```python
from build123d import *

# Parameters (mm, degrees)
F3_D = 15


with BuildPart() as f1:
    # F0 (on Right) → F1 (revolve)
    with BuildSketch(Plane.YZ):
        Polygon((-31.213203, 0), (0, 0), (0, 30), (-5, 30), (-15.606602, 19.393398), (-26.213203, 30), (-31.213203, 30), align=None)
    revolve(axis=Axis((0, -15.606602, 0), (0, 1, 0)))

    # F3 (through all)
    with Locations(Plane(origin=(0, 0, 0), x_dir=(1, 0, 0), z_dir=(0, 1, 0))):
        with Locations((0, 0)):
            Hole(F3_D / 2)


solid = f1.part
```
Work out the finished part from the listing and answer in its coordinate system (mm). Coordinates: 2 decimals unless noted, no trailing zeros. Order: outer loops, then holes, each group sorted by start corner. A loop starts at its lowest first (then second) coordinate and runs counter-clockwise, first axis right, second up. Notation, with made-up numbers: (87, 79) - (114, 79) arc R27 ccw to (114, 114) - close; hole circle Ø8 at (8.5, 44). An arc over 180 degrees is marked (long way). Answer as a JSON object with one key per item and string values.
1. Find section A-A on x = 0. Determine the outline of the cut face in (y, z).
Output values:
{"outline": "(-31.21, -30) - (-26.21, -30) - (-15.61, -19.39) - (-5, -30) - (0, -30) - (0, -7.5) - (-31.21, -7.5) - close; (-31.21, 7.5) - (0, 7.5) - (0, 30) - (-5, 30) - (-15.61, 19.39) - (-26.21, 30) - (-31.21, 30) - close"}
2. Find section B-B on z = 0. Determine the outline of the cut face in (x, y), plus the area to 3 significant figures.
Output values:
{"outline": "(-30, -31.21) - (-7.5, -31.21) - (-7.5, 0) - (-30, 0) - (-30, -5) - (-19.39, -15.61) - (-30, -26.21) - close; (7.5, -31.21) - (30, -31.21) - (30, -26.21) - (19.39, -15.61) - (30, -5) - (30, 0) - (7.5, 0) - close", "area": "1,180 mm²"}
3. Each of these flat-tipped pins is pushed along its axis until it touches: P1, Ø12, axis at y = -24.5, z = 20.5, coming from the -X side; P2, Ø1.5, axis at x = 11.5, y = -20.5, coming from the -Z side; P3, Ø1, axis at y = -27.5, z = -18.5, coming from the +X side; P4, Ø8, axis at x = -17.5, z = 10, coming from the +Y side. Where does it stop, or does it pass through?
Output values:
{"P1": "stops at x = -26.12", "P2": "stops at z = -22.32", "P3": "stops at x = 24", "P4": "stops at y = 0"}
4. Consider line 1 (Y direction, x = 8.5, z = 24.5); line 2 (Z direction, x = 0, y = -25); line 3 (Z direction, x = 0, y = -15). Determine where each line is inside the solid, lowest interval first.
Output values:
{"line 1": "y = -31.21 to -22.15, -9.07 to 0", "line 2": "z = -28.79 to -7.5, 7.5 to 28.79", "line 3": "z = -20 to -7.5, 7.5 to 20"}
5. The mould has two halves that part along Y. Classify faces 1 (the face through (-6, -31.213, 6)), 2 (the face through (-19.435, -15.092, -4.316)), 3 (the face through (1.32, -2.54, -29.97)), 4 (the face through (-19.58, -16.27, -4.35)): +Y half, -Y half, draft (parallel to the pull), parting line (faces both ways), or undercut.
Output values:
{"face 1": "-Y half", "face 2": "undercut", "face 3": "draft", "face 4": "undercut"}
6. Find section C-C on y = -2.5. Determine the outline of the cut face in (x, z), plus the area to 3 significant figures.
Output values:
{"outline": "circle Ø60 at (0, 0); hole circle Ø15 at (0, 0)", "area": "2,650 mm²"}
